from build123d import *

# Parameters (mm, degrees)
SKETCH1_W           = 70
SKETCH1_H           = 31.5
BOSS_EXTRUDE1_DEPTH = 8
SKETCH2_W           = 35
SKETCH2_H           = 8
BOSS_EXTRUDE2_DEPTH = 20
SKETCH3_R           = 2.6
CUT_EXTRUDE1_DEPTH  = 82.70832271
SKETCH4_W           = 49
SKETCH4_H           = 10
BOSS_EXTRUDE3_DEPTH = 10
SKETCH5_R           = 1.6
CUT_EXTRUDE2_DEPTH  = 82.70832271
SKETCH6_W           = 46
SKETCH6_H           = 9
CUT_EXTRUDE3_DEPTH  = 80.323703897
SKETCH7_R           = 5.6
CUT_EXTRUDE4_DEPTH  = 4
CUT_EXTRUDE5_START  = -4
SKETCH8_R           = 5.6
CUT_EXTRUDE5_DEPTH  = 4
SKETCH9_W           = 18
SKETCH9_H           = 6.5
CUT_EXTRUDE6_DEPTH  = 4
BOSS_EXTRUDE5_DEPTH = 20
CUT_EXTRUDE10_DEPTH = 5
BOSS_EXTRUDE6_DEPTH = 20
CUT_EXTRUDE11_DEPTH = 88.93747779
SKETCH17_W          = 49
SKETCH17_H          = 10
BOSS_EXTRUDE7_DEPTH = 10
SKETCH18_R          = 1.6
CUT_EXTRUDE12_DEPTH = 95.478833608
SKETCH19_W          = 35
SKETCH19_H          = 8
BOSS_EXTRUDE8_DEPTH = 20
SKETCH23_R          = 1.45
CUT_EXTRUDE13_DEPTH = 95.478833608
FILLET1_R           = 5


with BuildPart() as part:
    # Sketch1 → Boss-Extrude1 (new body)
    with BuildSketch(Plane(origin=(0, 0, 0), x_dir=(1, 0, 0), z_dir=(0, 1, 0))):
        with Locations((35, -15.75)):
            Rectangle(SKETCH1_W, SKETCH1_H)
    extrude(amount=BOSS_EXTRUDE1_DEPTH)

    # Sketch2 → Boss-Extrude2 (add)
    with BuildSketch(Plane(origin=(0, 8, 0), x_dir=(1, 0, 0), z_dir=(0, 1, 0))):
        with Locations((29.5, -27.5)):
            Rectangle(SKETCH2_W, SKETCH2_H)
        with Locations((29.5, -4)):
            Rectangle(SKETCH2_W, SKETCH2_H)
    extrude(amount=BOSS_EXTRUDE2_DEPTH)

    # Sketch3 → Cut-Extrude1 (cut, through all)
    with BuildSketch(Plane.XY.offset(31.5)):
        with Locations((30, 17)):
            Circle(SKETCH3_R)
    extrude(amount=-CUT_EXTRUDE1_DEPTH, mode=Mode.SUBTRACT)

    # Sketch4 → Boss-Extrude3 (add)
    with BuildSketch(Plane(origin=(0, 0, 0), x_dir=(-1, 0, 0), z_dir=(0, 0, -1))):
        with Locations((-24.5, 5)):
            Rectangle(SKETCH4_W, SKETCH4_H)
    extrude(amount=BOSS_EXTRUDE3_DEPTH)

    # Sketch5 → Cut-Extrude2 (cut, through all)
    with BuildSketch(Plane.ZY):
        with Locations((-5, 5)):
            Circle(SKETCH5_R)
    extrude(amount=-CUT_EXTRUDE2_DEPTH, mode=Mode.SUBTRACT)

    # Sketch6 → Cut-Extrude3 (cut, through all)
    with BuildSketch(Plane(origin=(0, 8, 0), x_dir=(1, 0, 0), z_dir=(0, 1, 0))):
        with Locations((30.25, -19)):
            Rectangle(SKETCH6_W, SKETCH6_H)
    extrude(amount=-CUT_EXTRUDE3_DEPTH, mode=Mode.SUBTRACT)

    # Sketch7 → Cut-Extrude4 (cut)
    with BuildSketch(Plane.XY.offset(8)):
        with Locations((30, 17)):
            Circle(SKETCH7_R)
    extrude(amount=-CUT_EXTRUDE4_DEPTH, mode=Mode.SUBTRACT)

    # Sketch8 → Cut-Extrude5 (cut)
    with BuildSketch(Plane(origin=(0, 0, 23.5), x_dir=(-1, 0, 0), z_dir=(0, 0, -1)).offset(CUT_EXTRUDE5_START)):
        with Locations(Location((-30, 17, 0), (0, 0, 180))):
            Circle(SKETCH8_R)
    extrude(amount=CUT_EXTRUDE5_DEPTH, mode=Mode.SUBTRACT)

    # Sketch9 → Cut-Extrude6 (cut)
    with BuildSketch(Plane(origin=(0, 8, 0), x_dir=(1, 0, 0), z_dir=(0, 1, 0))):
        with Locations((30, -11.25)):
            Rectangle(SKETCH9_W, SKETCH9_H)
    extrude(amount=-CUT_EXTRUDE6_DEPTH, mode=Mode.SUBTRACT)

    # Sketch13 → Boss-Extrude5 (add)
    with BuildSketch(Plane(origin=(0, 8, 0), x_dir=(1, 0, 0), z_dir=(0, 1, 0))):
        Polygon((70, -13), (43, -13), (43, -8), (47, -8), (47, -5), (70, -5), align=None)
    extrude(amount=BOSS_EXTRUDE5_DEPTH)

    # Sketch14 → Cut-Extrude10 (cut)
    with BuildSketch(Plane(origin=(0, 0, 0), x_dir=(-1, 0, 0), z_dir=(0, 0, -1))):
        Polygon((-33.697877871, 28), (-40.874528252, 10), (-47, 10), (-47, 28), align=None)
    extrude(amount=-CUT_EXTRUDE10_DEPTH, mode=Mode.SUBTRACT)

    # Sketch15 → Boss-Extrude6 (add)
    with BuildSketch(Plane(origin=(0, 28, 0), x_dir=(1, 0, 0), z_dir=(0, 1, 0))):
        Polygon((70, -5), (70, -13), (43, -13), (43, -8), (33.697877871, -8), (24.157827733, -8), (12, -8), (12, 0), (24.157827733, 0), (33.697877871, 0), (33.697877871, -5), align=None)
    extrude(amount=BOSS_EXTRUDE6_DEPTH)

    # Sketch16 → Cut-Extrude11 (cut, through all)
    with BuildSketch(Plane.XY.offset(13)):
        with BuildLine():
            Line((52.5, 37.5), (58.5, 37.5))
            ThreePointArc((58.5, 37.5), (65, 31), (58.5, 24.5))
            Line((58.5, 24.5), (52.5, 24.5))
            ThreePointArc((52.5, 24.5), (46, 31), (52.5, 37.5))
        make_face()
        with BuildLine():
            Line((52.5, 45.1), (58.5, 45.1))
            ThreePointArc((58.5, 45.1), (60.1, 43.5), (58.5, 41.9))
            Line((58.5, 41.9), (52.5, 41.9))
            ThreePointArc((52.5, 41.9), (50.9, 43.5), (52.5, 45.1))
        make_face()
        with BuildLine():
            Line((52.5, 20.1), (58.5, 20.1))
            ThreePointArc((58.5, 20.1), (60.1, 18.5), (58.5, 16.9))
            Line((58.5, 16.9), (52.5, 16.9))
            ThreePointArc((52.5, 16.9), (50.9, 18.5), (52.5, 20.1))
        make_face()
    extrude(amount=-CUT_EXTRUDE11_DEPTH, mode=Mode.SUBTRACT)

    # Sketch17 → Boss-Extrude7 (add)
    with BuildSketch(Plane.XY.offset(31.5)):
        with Locations((24.5, 5)):
            Rectangle(SKETCH17_W, SKETCH17_H)
    extrude(amount=BOSS_EXTRUDE7_DEPTH)

    # Sketch18 → Cut-Extrude12 (cut, through all)
    with BuildSketch(Plane.ZY):
        with Locations((36.5, 5)):
            Circle(SKETCH18_R)
    extrude(amount=-CUT_EXTRUDE12_DEPTH, mode=Mode.SUBTRACT)

    # Sketch19 → Boss-Extrude8 (add)
    with BuildSketch(Plane(origin=(0, 28, 0), x_dir=(1, 0, 0), z_dir=(0, 1, 0))):
        with Locations((29.5, -27.5)):
            Rectangle(SKETCH19_W, SKETCH19_H)
    extrude(amount=BOSS_EXTRUDE8_DEPTH)

    # Sketch23 → Cut-Extrude13 (cut, through all)
    with BuildSketch(Plane(origin=(0, 48, 0), x_dir=(1, 0, 0), z_dir=(0, 1, 0))):
        with Locations(Location((16, -27.5, 0), (0, 0, 270))):
            Circle(SKETCH23_R)
        with Locations(Location((16, -4, 0), (0, 0, 270))):
            Circle(SKETCH23_R)
        with Locations(Location((22, -27.5, 0), (0, 0, 270))):
            Circle(SKETCH23_R)
        with Locations(Location((22, -4, 0), (0, 0, 270))):
            Circle(SKETCH23_R)
    extrude(amount=-CUT_EXTRUDE13_DEPTH, mode=Mode.SUBTRACT)

    # Fillet1
    fillet1_edges = [part.edges().sort_by_distance(p)[0] for p in [
        (24.5, 10, 41.5),
        (24.5, 10, -10),
    ]]
    fillet(fillet1_edges, radius=FILLET1_R)


solid = part.part
Verification items for the finished model (mm, model axes). A direction names the side the tool comes from. Coordinates: 2 decimals unless noted, no trailing zeros. Order: outer loops, then holes, each group sorted by start corner. A loop starts at its lowest first (then second) coordinate and runs counter-clockwise, first axis right, second up.
Item 1: Section check B-B, the plane y = 43.5. Enter the section's corners in (x, z), then the cut area to 3 significant figures.
Filled in:
outline: (12, 0) - (33.7, 0) - (33.7, 5) - (50.9, 5) - (50.9, 13) - (43, 13) - (43, 8) - (12, 8) - close; (12, 23.5) - (47, 23.5) - (47, 31.5) - (12, 31.5) - close; (60.1, 5) - (70, 5) - (70, 13) - (60.1, 13) - close; hole circle Ø2.9 at (16, 4); hole circle Ø2.9 at (16, 27.5); hole circle Ø2.9 at (22, 4); hole circle Ø2.9 at (22, 27.5)
area: 597 mm2
Item 2: Access from +Z, -Z, +X, -X, +Y, -Y to the whole of each face (thin tool, end or side, straight path). Record for faces 1 (the face through (24, 10, 34)), 2 (the face through (55, 37.5, 9)), 3 (the face through (25.56, 20.41, 25.53)).
Filled in:
face 1: +Z, +X, -X, +Y
face 2: +Z, -Z
face 3: none
Item 3: Release check for a two-part mould opening along Y. For faces 4 (the face through (20.714, 24.336, 28.169)), 5 (the face through (24, 8, -9)), 6 (the face through (50.9, 43.5, 9.1)) record: +Y half, -Y half, draft (parallel to the pull), parting line (faces both ways), or undercut.
Filled in:
face 4: draft
face 5: +Y half
face 6: undercut
Item 4: Section check A-A, the plane x = 16. Enter the section's corners in (y, z), then the cut area to 3 significant figures.
Filled in:
outline: (0, -10) - (5, -10) arc R5 ccw to (10, -5) - (10, 0) - (48, 0) - (48, 2.55) - (0, 2.55) - close; (0, 5.45) - (48, 5.45) - (48, 8) - (8, 8) - (8, 14.5) - (0, 14.5) - close; (0, 23.5) - (48, 23.5) - (48, 26.05) - (0, 26.05) - close; (0, 28.95) - (48, 28.95) - (48, 31.5) - (10, 31.5) - (10, 36.5) arc R5 ccw to (5, 41.5) - (0, 41.5) - close; hole circle Ø3.2 at (5, -5); hole circle Ø3.2 at (5, 36.5)
area: 715 mm2
Item 5: Material ranges on L1, parallel to X at y = 11, z = 27.5; L2, parallel to Z at x = 19, y = 28.5; L3, parallel to Z at x = 36.5, y = 41.5, recorded low to high.
Filled in:
L1: x = 12 to 14.55, 17.45 to 20.55, 23.45 to 47
L2: z = 0 to 8, 23.5 to 31.5
L3: z = 5 to 8, 23.5 to 31.5
Item 6: Section check C-C, the plane z = 21. Enter the section's corners in (x, y), then the cut area to 3 significant figures.
Filled in:
outline: (0, 0) - (7.25, 0) - (7.25, 8) - (0, 8) - close; (53.25, 0) - (70, 0) - (70, 8) - (53.25, 8) - close
area: 192 mm2
Item 7: Depth check by flat-ended pin: pin 1 (2 mm diameter, centred on y = 40.5, z = -2.5, fed in from -X); pin 2 (23 mm diameter, centred on x = 26, y = 36, fed in from -Z); pin 3 (12 mm diameter, centred on y = 18.5, z = 33.5, fed in from -X); pin 4 (1 mm diameter, centred on y = 9.5, z = 3, fed in from +X). Enter the tip coordinate at first touch or a pass-through.
Filled in:
pin 1: passes through
pin 2: stops at z = 0
pin 3: stops at x = 12
pin 4: stops at x = 47
Item 8: Section check D-D, the plane y = 21. Enter the section's corners in (x, z), then the cut area to 3 significant figures.
Filled in:
outline: (12, 0) - (36.49, 0) - (36.49, 5) - (70, 5) - (70, 13) - (43, 13) - (43, 8) - (33.92, 8) - (33.92, 4) - (26.08, 4) - (26.08, 8) - (12, 8) - close; (12, 23.5) - (26.08, 23.5) - (26.08, 27.5) - (33.92, 27.5) - (33.92, 23.5) - (47, 23.5) - (47, 31.5) - (12, 31.5) - close; hole circle Ø2.9 at (16, 4); hole circle Ø2.9 at (16, 27.5); hole circle Ø2.9 at (22, 4); hole circle Ø2.9 at (22, 27.5)
area: 622 mm2
